Autodesk Fusion 360 part; units mm, degrees
sketch "Sketch1" plane through (0, 0, 0) normal (0, 0, 1) x (1, 0, 0)
  line L0 (-28.5, -24) -> (-28.5, 24)
  line L1 (-28.5, 24) -> (28.5, 24)
  line L2 (28.5, 24) -> (28.5, -24)
  line L3 (-28.5, -24) -> (28.5, -24)
  circle A0 centre (-28.5, 24) radius 1.5
  circle A1 centre (28.5, 24) radius 1.5
  circle A2 centre (-28.5, -24) radius 1.5
  circle A3 centre (28.5, -24) radius 1.5
  line L4 (0, 24) -> (0, -24)
  line L5 (0, 0) -> (-28.5, 0)
  line L6 (-31.5, -27) -> (31.5, -27)
  line L7 (31.5, 27) -> (31.5, -27)
  line L8 (-31.5, 27) -> (31.5, 27)
  line L9 (-31.5, -27) -> (-31.5, 27)
  dimension "d1" = 3
  dimension "d2" = 3
  dimension "d3" = 3
  dimension "d4" = 3
  dimension "d5" = -3
extrude "Extrude1" add sketch "Sketch1" along normal blind 3 contours L0 L3 A2 L4 L5 | L0 L1 A0 L4 L5 | L1 L2 L3 A1 A3 L4 | L6 L7 L8 L9
sketch "Sketch2" plane through (0, 0, 3) normal (0, 0, 1) x (-1, 0, 0)
  circle A0 centre (-28.5, -24) radius 1.5
  circle A1 centre (28.5, 24) radius 1.5
  circle A2 centre (28.5, -24) radius 1.5
  circle A3 centre (-28.5, 24) radius 1.5
  line L0 (31.5, 27) -> (-31.5, 27)
  line L1 (-31.5, 27) -> (-31.5, -27)
  line L2 (-31.5, -27) -> (31.5, -27)
  line L3 (31.5, -27) -> (31.5, 27)
  line L4 (-15, -19.5) -> (15, -19.5)
  line L5 (12, -14.5) -> (-12, -14.5)
  circle A4 centre (14, -16.5) radius 1.5
  line L6 (15, -19.5) -> (17, -17.5)
  line L7 (17, -17.5) -> (17, 0)
  line L8 (17, 0) -> (12, 0)
  line L9 (12, 0) -> (12, -14.5)
  line L10 (-12, -14.5) -> (-12, 0)
  line L11 (-12, 0) -> (-17, 0)
  line L12 (-17, 0) -> (-17, -17.5)
  line L13 (-17, -17.5) -> (-15, -19.5)
  circle A5 centre (-14, -16.5) radius 1.5
  line L14 (12, 0) -> (-12, 0)
  line L15 (0, 0) -> (0, -7.25)
  line L16 (12, 0) -> (12, 14.5)
  line L17 (17, 17.5) -> (17, 0)
  line L18 (17, 0) -> (12, 0)
  line L19 (-15, 19.5) -> (15, 19.5)
  line L20 (12, 14.5) -> (-12, 14.5)
  line L21 (-12, 14.5) -> (-12, 0)
  circle A6 centre (14, 16.5) radius 1.5
  circle A7 centre (-14, 16.5) radius 1.5
  line L22 (-17, 17.5) -> (-15, 19.5)
  line L23 (-17, 0) -> (-17, 17.5)
  line L24 (-12, 0) -> (-17, 0)
  line L25 (15, 19.5) -> (17, 17.5)
extrude "Extrude2" add sketch "Sketch2" along normal blind 90 contours L4 L5 L6 L7 L8 L9 L10 L11 L12 L13 L18 L24 | L8 L11 L16 L17 L18 L19 L20 L21 L22 L23 L24 L25
fillet "Fillet1" radius 3 4 edges at (-31.5, -27, 1.5) (31.5, -27, 1.5) (31.5, 27, 1.5) (-31.5, 27, 1.5)
fillet "Fillet2" radius 2.5 8 edges at (30.6213, 26.1213, 3) (0, 27, 3) (-30.6213, 26.1213, 3) (-31.5, 0, 3) (-30.6213, -26.1213, 3) (0, -27, 3) (30.6213, -26.1213, 3) (31.5, 0, 3)
chamfer "Chamfer1" distance 3 angle 45 8 edges at (0, 19.5, 3) (17, 0, 3) (16, 18.5, 3) (-16, 18.5, 3) (-16, -18.5, 3) (-17, 0, 3) (0, -19.5, 3) (16, -18.5, 3)
sketch "Sketch3" plane through (0, 19.5, 0) normal (0, 1, 0) x (-1, 0, 0)
  line L0 (15, 6) -> (15, 93)
  line L1 (15, 93) -> (-15, 93)
  line L2 (-15, 93) -> (-15, 6)
  line L3 (-15, 49.5) -> (15, 49.5)
  circle A0 centre (0, 49.5) radius 9.5
  line L4 (-15, 6) -> (15, 6)
  dimension "d12" = 19
extrude "Extrude3" cut sketch "Sketch3" against normal blind 6 contours L3 A0 | L3 A0
sketch "Sketch4" plane through (0, 0, 93) normal (0, 0, 1) x (-1, 0, 0)
  circle A0 centre (14, -16.5) radius 1.5
  circle A1 centre (14, 16.5) radius 1.5
  circle A2 centre (-14, -16.5) radius 1.5
  line L0 (12, 14.5) -> (12, -14.5)
  line L1 (12, -14.5) -> (-12, -14.5)
  line L2 (-12, -14.5) -> (-12, 14.5)
  line L3 (-12, 14.5) -> (12, 14.5)
  circle A3 centre (-14, 16.5) radius 1.5
  line L4 (-17, 17.5) -> (-17, -17.5)
  line L5 (-17, -17.5) -> (-15, -19.5)
  line L6 (-15, -19.5) -> (15, -19.5)
  line L7 (15, -19.5) -> (17, -17.5)
  line L8 (17, -17.5) -> (17, 17.5)
  line L9 (17, 17.5) -> (15, 19.5)
  line L10 (15, 19.5) -> (-15, 19.5)
  line L11 (-15, 19.5) -> (-17, 17.5)
  line L12 (-50, 0) -> (50, 0)
  line L13 (50, 0) -> (33.9234, 54.6299)
  line L14 (33.9234, 54.6299) -> (-46.2592, 44.9375)
  line L15 (-46.2592, 44.9375) -> (-50, 0)
  line L16 (12, 14.5) -> (-12, 14.5)
  line L17 (-12, 14.5) -> (-12, -14.5)
  line L18 (-12, -14.5) -> (12, -14.5)
  line L19 (12, -14.5) -> (12, 14.5)
  line L20 (-50, 0) -> (-64.2202, -68.1179)
  line L21 (-64.2202, -68.1179) -> (43.9074, -45.7813)
  line L22 (43.9074, -45.7813) -> (50, 0)
extrude "Extrude4" cut sketch "Sketch4" against normal blind 500 contours A0 | A2 | L0 L2 L3 L12 L16 L17 L19 | L0 L1 L2 L4 L5 L6 L7 L8 L12 L17 L18 L19 | L0 L1 L2 L12 L17 L18 L19 | L4 L5 L6 L7 L8 L12 L20 L21 L22
Design review of the part built by this model. Coordinates are the model's own, in mm. A direction names the side the tool comes from. Round coordinates to 2 decimals unless told otherwise and drop trailing zeros. Write each loop counter-clockwise with the first axis right and the second up, starting at its lowest first coordinate (ties: lowest second). Pieces come first, ordered by that corner, then holes. Notation, with made-up numbers: (79.5, -6.75) -> (86.5, -6.75) arc R23 ccw to (86.5, 10.25) -> close; hole circle Ø3 at (55.5, 2.25). An arc over 180 degrees is marked (long way). One line per item, written item: value. Start each with the question number.
Q1. Tool access review of faces 4 (the face through (17, -9, 49)), 5 (the face through (15.5, -16.43, 47.37)), 6 (the face through (-17, -9, 49)), 7 (the face through (16, -18.5, 48.9)), 8 (the face through (-12, -7, 47)): name each direction out of +Z, -Z, +X, -X, +Y, -Y from which nothing blocks a thin tool from reaching the whole face with its end or side.
Q2. Add section B-B (x = 3). Give the boundary of the cut face in (y, z), then the cut area to 3 significant figures.
Q3. The part is to be moulded in two halves that separate along Y. For faces 1 (the face through (12, -7, 46)), 2 (the face through (-16, -18.5, 48.9)), 3 (the face through (14, -16, 3)), say which applies: pulls with the +Y half, pulls with the -Y half, needs draft (parallel to the pull), parting line crosses it, or undercut.
Q4. Add section D-D (y = -16.5). Give the boundary of the cut face in (x, z).
Q5. Add section A-A (y = -3.5). Give the boundary of the cut face in (x, z), then the cut area to 3 significant figures.
Q6. Add section C-C (z = 18). Give the boundary of the cut face in (x, y).
Q7. To check wall thickness, follow probe 1 along X at (y, z) = (-24, 1.05); probe 2 along X at (y, z) = (-16.5, 64); probe 3 along X at (y, z) = (-4.5, 81). State the ranges of each line that lie inside material, in increasing order.
Q8. Insertion check: P1, Ø0.9, axis at x = -14.5, y = -16, coming from the +Z side; P2, Ø11.5, axis at y = -6.5, z = 65.5, coming from the +X side; P3, Ø3, axis at x = -14.5, z = 23.5, coming from the +Y side; P4, Ø4.5, axis at y = -7.5, z = 40.5, coming from the -X side. Each pin has a flat end and moves straight along its axis. Give the tip position at first contact, or say it passes through.
Response:
1. face 4: +Z, +X, +Y, -Y
1. face 5: +Z
1. face 6: +Z, -X, +Y, -Y
1. face 7: +Z, +X, -Y
1. face 8: +Z, -Z, +Y
2. outline: (-27, 0) -> (-14.5, 0) -> (-14.5, 93) -> (-19.5, 93) -> (-19.5, 6) -> (-22.5, 3) -> (-24.5, 3) arc R2.5 ccw to (-27, 0.5) -> close
2. area: 491 mm^2
3. face 1: needs draft
3. face 2: pulls with the -Y half
3. face 3: undercut
4. outline: (-31.5, 0) -> (31.5, 0) -> (31.5, 0.5) arc R2.5 ccw to (29, 3) -> (20, 3) -> (17, 6) -> (17, 93) -> (15.5, 93) -> (15.5, 3) -> (12.5, 3) -> (12.5, 93) -> (-12.5, 93) -> (-12.5, 3) -> (-15.5, 3) -> (-15.5, 93) -> (-17, 93) -> (-17, 6) -> (-20, 3) -> (-29, 3) arc R2.5 ccw to (-31.5, 0.5) -> close
5. outline: (-31.5, 0) -> (-12, 0) -> (-12, 93) -> (-17, 93) -> (-17, 6) -> (-20, 3) -> (-29, 3) arc R2.5 ccw to (-31.5, 0.5) -> close; (12, 0) -> (31.5, 0) -> (31.5, 0.5) arc R2.5 ccw to (29, 3) -> (20, 3) -> (17, 6) -> (17, 93) -> (12, 93) -> close
5. area: 1,020 mm^2
6. outline: (-17, -17.5) -> (-15, -19.5) -> (15, -19.5) -> (17, -17.5) -> (17, 0) -> (12, 0) -> (12, -14.5) -> (-12, -14.5) -> (-12, 0) -> (-17, 0) -> close; hole circle Ø3 at (-14, -16.5); hole circle Ø3 at (14, -16.5)
7. probe 1: x = -31.48 to -30, -27 to 27, 30 to 31.48
7. probe 2: x = -17 to -15.5, -12.5 to 12.5, 15.5 to 17
7. probe 3: x = -17 to -12, 12 to 17
8. P1: stops at z = 3
8. P2: stops at x = 17
8. P3: stops at y = 0
8. P4: stops at x = -17
